Work out the finished part from the listing and answer in its coordinate system (mm). A direction names the side the tool comes from. Coordinates: 2 decimals unless noted, no trailing zeros. Loops run counter-clockwise (first coordinate to the right, second up) from the corner with the lowest first, then second, coordinate; pieces in that order, holes last. Notation, with made-up numbers: (-3, 89.25) - (28, 89.25) arc R21 cw to (28, 109.25) - close; hole circle Ø7 at (-18, 82.25). An arc over 180 degrees is marked (long way). Write each question's results on one line, items separated by ' | '. Start each with the question number.
Item 1: A tool of negligible diameter and unlimited length cuts with its end or side. For faces 4 (the face through (-40, 0, 0)), 5 (the face through (-24.1, -9.14, -0.15)), from which of +Z, -Z, +X, -X, +Y, -Y can it reach the whole face along a straight path? Write none if from no direction.
Item 2: For a pull along Y with two mould halves and no side action, classify faces 1 (the face through (40, 0, 0)), 2 (the face through (0, 15, 0)), 3 (the face through (-31.548, 6.919, 0.154)) as +Y half, -Y half, draft (parallel to the pull), parting line (faces both ways), or undercut.
Item 3: Section C-C, the plane z = 9.25 is taken. Write down the section's boundary in (x, y), plus the area to 3 significant figures.
Item 4: Section D-D, the plane x = 4 is taken. Write down the section's boundary in (y, z), plus the area to 3 significant figures.
Item 5: Section A-A, the plane y = 5.5 is taken. Write down the section's boundary in (x, z), plus the area to 3 significant figures.
Item 6: This flat-tipped pin is pushed along its axis until it touches: pin 1 Ø2.5 at (x, y) = (30, 5.5) entering from -Z. Where does it stop, or does it pass through?
Item 7: Section B-B, the plane x = 30 is taken. Write down the section's boundary in (y, z).
Item 8: Consider probe 1 along Y at (x, z) = (30, 3.75); probe 2 along Y at (x, z) = (-3, 8); probe 3 along X at (y, z) = (-0.75, -8.5). Determine where each line is inside the solid, lowest interval first. Write a range as [from, to].
from build123d import *

# Parameters (mm, degrees)
SKETCH_1_W          = 80
SKETCH_1_H          = 30
EXTRUDE_1_DEPTH     = 11
FILLET_1_R          = 5
SKETCH_2_R          = 2.1
SKETCH_2_W          = 50
SKETCH_2_H          = 20
CUT_EXTRUDE_1_DEPTH = 23
FILLET_2_R          = 3


with BuildPart() as part:
    # 草图1 → 凸台-拉伸1 (new body, symmetric)
    with BuildSketch(Plane.XY):
        Rectangle(SKETCH_1_W, SKETCH_1_H)
    extrude(amount=EXTRUDE_1_DEPTH, both=True)

    # 圆角1
    fillet_1_edges = [part.edges().sort_by_distance(p)[0] for p in [
        (40, -15, 0),
        (-40, -15, 0),
        (-40, 15, 0),
        (40, 15, 0),
    ]]
    fillet(fillet_1_edges, radius=FILLET_1_R)

    # 草图2 → 切除-拉伸1 (cut, through all)
    with BuildSketch(Plane.XY.offset(11)):
        with Locations((-30, 5.5)):
            Circle(SKETCH_2_R)
        with Locations((30, 5.5)):
            Circle(SKETCH_2_R)
        with Locations((30, -9.5)):
            Circle(SKETCH_2_R)
        with Locations((-30, -9.5)):
            Circle(SKETCH_2_R)
        Rectangle(SKETCH_2_W, SKETCH_2_H)
    extrude(amount=-CUT_EXTRUDE_1_DEPTH, mode=Mode.SUBTRACT)

    # 圆角2
    fillet_2_edges = [part.edges().sort_by_distance(p)[0] for p in [
        (25, 10, 0),
        (25, -10, 0),
        (-25, -10, 0),
        (-25, 10, 0),
    ]]
    fillet(fillet_2_edges, radius=FILLET_2_R)


solid = part.part
Answer key:
1) face 4: +Z, -Z, -X, +Y, -Y | face 5: +Z, -Z
2) face 1: draft | face 2: +Y half | face 3: undercut
3) outline: (-40, -10) arc R5 ccw to (-35, -15) - (35, -15) arc R5 ccw to (40, -10) - (40, 10) arc R5 ccw to (35, 15) - (-35, 15) arc R5 ccw to (-40, 10) - close; hole circle Ø4.2 at (-30, -9.5); hole circle Ø4.2 at (-30, 5.5); hole (-25, -7) arc R3 ccw to (-22, -10) - (22, -10) arc R3 ccw to (25, -7) - (25, 7) arc R3 ccw to (22, 10) - (-22, 10) arc R3 ccw to (-25, 7) - close; hole circle Ø4.2 at (30, -9.5); hole circle Ø4.2 at (30, 5.5) | area: 1,330 mm^2
4) outline: (-15, -11) - (-10, -11) - (-10, 11) - (-15, 11) - close; (10, -11) - (15, -11) - (15, 11) - (10, 11) - close | area: 220 mm^2
5) outline: (-40, -11) - (-32.1, -11) - (-32.1, 11) - (-40, 11) - close; (-27.9, -11) - (-25, -11) - (-25, 11) - (-27.9, 11) - close; (25, -11) - (27.9, -11) - (27.9, 11) - (25, 11) - close; (32.1, -11) - (40, -11) - (40, 11) - (32.1, 11) - close | area: 475 mm^2
6) pin 1: passes through
7) outline: (-15, -11) - (-11.6, -11) - (-11.6, 11) - (-15, 11) - close; (-7.4, -11) - (3.4, -11) - (3.4, 11) - (-7.4, 11) - close; (7.6, -11) - (15, -11) - (15, 11) - (7.6, 11) - close
8) probe 1: y = [-15, -11.6], [-7.4, 3.4], [7.6, 15] | probe 2: y = [-15, -10], [10, 15] | probe 3: x = [-40, -25], [25, 40]
